```python
from build123d import *

# Parameters (mm, degrees)
SKETCH_1_W           = 76.5
SKETCH_1_H           = 50.4
SKETCH_1_W_2         = 72.5
SKETCH_1_H_2         = 46.4
EXTRUDE_1_DEPTH      = 3
SKETCH_2_W           = 26.5
SKETCH_2_H           = 2
SKETCH_2_W_2         = 2
SKETCH_2_H_2         = 7
EXTRUDE_2_DEPTH      = 3
EXTRUDE_4_DEPTH      = 2
EXTRUDE_4_DEPTH_BACK = 18
SKETCH_3_W           = 76.541364071
SKETCH_3_H           = 20
SKETCH_3_R           = 2.7
FILLET_1_R           = 3
CUT_EXTRUDE_1_DEPTH  = 18
SKETCH_5_W           = 42.5
SKETCH_5_H           = 5
EXTRUDE_5_DEPTH      = 2
EXTRUDE_6_DEPTH      = 2
SKETCH_7_W           = 26.5
SKETCH_7_H           = 2
EXTRUDE_7_DEPTH      = 2
SKETCH_8_W           = 67.5
SKETCH_8_H           = 2
EXTRUDE_8_DEPTH      = 10


with BuildPart() as part:
    # 草图1 → 凸台-拉伸1 (new body)
    with BuildSketch(Plane(origin=(0, 0, 0), x_dir=(0, 0, -1), z_dir=(1, 0, 0))):
        with Locations((36.25, 23.2)):
            Rectangle(SKETCH_1_W, SKETCH_1_H)
        with Locations((36.25, 23.2)):
            Rectangle(SKETCH_1_W_2, SKETCH_1_H_2, mode=Mode.SUBTRACT)
    extrude(amount=EXTRUDE_1_DEPTH)

    # 草图2 → 凸台-拉伸2 (add)
    with BuildSketch(Plane(origin=(3, 0, 0), x_dir=(0, 0, -1), z_dir=(1, 0, 0))):
        with Locations((36.25, -1)):
            Rectangle(SKETCH_2_W, SKETCH_2_H)
        Polygon((-2, -2), (0, -2), (5, -2), (5, 0), (0, 0), (0, 28), (-2, 28), align=None)
        Polygon((74.5, -2), (72.5, -2), (67.5, -2), (67.5, 0), (72.5, 0), (72.5, 8), (74.5, 8), align=None)
        Polygon((-2, 48.4), (5, 48.4), (5, 46.4), (0, 46.4), (0, 41.4), (-2, 41.4), (-2, 46.4), align=None)
        with Locations((73.5, 44.9)):
            Rectangle(SKETCH_2_W_2, SKETCH_2_H_2)
    extrude(amount=EXTRUDE_2_DEPTH)

    # 草图3 → 凸台-拉伸4 (add, two sides: drawn at the far end of the back side and taken through both)
    with BuildSketch(Plane.ZY.offset(-EXTRUDE_4_DEPTH_BACK)):
        with Locations((-36.229317964, 58.4)):
            Rectangle(SKETCH_3_W, SKETCH_3_H)
        with Locations((-59.5, 53.4)):
            Circle(SKETCH_3_R, mode=Mode.SUBTRACT)
        with Locations((-12.958635929, 53.4)):
            Circle(SKETCH_3_R, mode=Mode.SUBTRACT)
        with Locations((-34.458635929, 53.4)):
            Circle(SKETCH_3_R, mode=Mode.SUBTRACT)
    extrude(amount=EXTRUDE_4_DEPTH + EXTRUDE_4_DEPTH_BACK)

    # 圆角1
    fillet_1_edges = [part.edges().sort_by_distance(p)[0] for p in [
        (18, 68.4, -36.229317964),
    ]]
    fillet(fillet_1_edges, radius=FILLET_1_R)

    # 草图4 → 切除-拉伸1 (cut)
    with BuildSketch(Plane(origin=(0, 68.4, 0), x_dir=(1, 0, 0), z_dir=(0, 1, 0))):
        with BuildLine():
            Line((7.8, 66.5), (7.8, 51.5))
            ThreePointArc((7.8, 51.5), (5.15, 48.85), (2.5, 51.5))
            Line((2.5, 51.5), (2.5, 66.5))
            ThreePointArc((2.5, 66.5), (5.15, 69.15), (7.8, 66.5))
        make_face()
        with BuildLine():
            Line((7.8, 29.958635929), (7.8, 9.958635929))
            ThreePointArc((7.8, 9.958635929), (5.15, 7.308635929), (2.5, 9.958635929))
            Line((2.5, 9.958635929), (2.5, 29.958635929))
            ThreePointArc((2.5, 29.958635929), (5.15, 32.608635929), (7.8, 29.958635929))
        make_face()
    extrude(amount=-CUT_EXTRUDE_1_DEPTH, mode=Mode.SUBTRACT)

    # 草图5 → 凸台-拉伸5 (add)
    with BuildSketch(Plane.ZY):
        Polygon((-35.66479448, 48.4), (-36.83520552, 48.4), (-57.5, 35.174531533), (-57.5, 48.4), (-60.5, 48.4), (-60.5, 33.254531533), (-74.5, 24.294531533), (-74.5, 21.2), (2, 21.2), (2, 24.294531533), (-12, 33.254531533), (-12, 48.4), (-15, 48.4), (-15, 35.174531533), align=None)
        Polygon((-60.5, 23.2), (-72.5, 23.2), (-60.5, 30.88), align=None, mode=Mode.SUBTRACT)
        with Locations((-36.25, 25.7)):
            Rectangle(SKETCH_5_W, SKETCH_5_H, mode=Mode.SUBTRACT)
        Polygon((-12, 30.88), (0, 23.2), (-12, 23.2), align=None, mode=Mode.SUBTRACT)
        Polygon((-57.5, 32.8), (-36.25, 46.4), (-15, 32.8), (-15, 30.88), (-57.5, 30.88), align=None, mode=Mode.SUBTRACT)
    extrude(amount=EXTRUDE_5_DEPTH)

    # 草图6 → 凸台-拉伸6 (add)
    with BuildSketch(Plane.ZY):
        Polygon((0, 46.4), (0, 25.574531533), (2, 24.294531533), (2, 48.4), (-12, 48.4), (-12, 46.4), align=None)
        Polygon((-74.5, 48.4), (-74.5, 24.294531533), (-72.5, 25.574531533), (-72.5, 46.4), (-60.5, 46.4), (-60.5, 48.4), align=None)
        Polygon((2, -2), (2, 21.2), (0, 21.2), (0, 0), (-72.5, 0), (-72.5, 21.2), (-74.5, 21.2), (-74.5, -2), align=None)
        Polygon((-15, 46.4), (-15, 48.4), (-35.66479448, 48.4), (-32.53979448, 46.4), align=None)
        Polygon((-57.5, 46.4), (-39.96020552, 46.4), (-36.83520552, 48.4), (-57.5, 48.4), align=None)
    extrude(amount=EXTRUDE_6_DEPTH)

    # 草图7 → 凸台-拉伸7 (add)
    with BuildSketch(Plane(origin=(6, 0, 0), x_dir=(0, 0, -1), z_dir=(1, 0, 0))):
        with Locations((36.25, -1)):
            Rectangle(SKETCH_7_W, SKETCH_7_H)
    extrude(amount=EXTRUDE_7_DEPTH)

    # 草图8 → 凸台-拉伸8 (add)
    with BuildSketch(Plane(origin=(3, 0, 0), x_dir=(0, 0, -1), z_dir=(1, 0, 0))):
        with Locations((38.75, 47.4)):
            Rectangle(SKETCH_8_W, SKETCH_8_H)
    extrude(amount=EXTRUDE_8_DEPTH)


solid = part.part
```
The listing builds one solid part. Answer for the finished solid, in the listing's coordinates (mm). A direction names the side the tool comes from. Give positions to 0.01 mm unless a question says otherwise; leave off trailing zeros. Loops run counter-clockwise (first coordinate to the right, second up) from the corner with the lowest first, then second, coordinate; pieces in that order, holes last. Notation, with made-up numbers: M -23,37 L 10,37 A14 cw 10,62 Z; hole C 32,22.25 d3. An arc over 180 degrees is marked long. One line per item, written item: value.
1. Section C-C on x = 1.25 is taken. Determine the outline of the cut face in (y, z).
Found:
outline: M -2,-74.5 L 68.4,-74.5 L 68.4,2.04 L 48.4,2.04 L 48.4,2 L -2,2 Z; hole M 0,-72.5 L 46.4,-72.5 L 46.4,0 L 0,0 Z; hole C 53.4,-59.5 d5.4; hole C 53.4,-34.46 d5.4; hole C 53.4,-12.96 d5.4
2. For a pull along Y with two mould halves and no side action, classify faces 5 (the face through (5.21, 59.53, -7.31)), 6 (the face through (0, 30, -34)), 7 (the face through (7, 68.4, -37)) as pulls with the +Y half, pulls with the -Y half, needs draft (parallel to the pull), parting line crosses it, or undercut.
Found:
face 5: needs draft
face 6: undercut
face 7: pulls with the +Y half
3. Each of these flat-tipped pins is pushed along its axis until it touches: P1, Ø12, axis at x = 15, z = -22.5, coming from the -Y side; P2, Ø1, axis at x = 8, y = 47.5, coming from the +Z side; P3, Ø0.6, axis at y = 33.5, z = 1.5, coming from the +X side; P4, Ø1.5, axis at y = 19, z = -36, coming from the +X side. Where does it stop, or does it pass through?
Found:
P1: y = 46.4
P2: z = -5
P3: x = 3
P4: through
4. Find the intervals of material crossed by probe 1 along Y at (x, z) = (11, -59.5); probe 2 along Z at (x, y) = (6.5, 53); probe 3 along Y at (x, z) = (-0.5, -59), in increasing order.
Found:
probe 1: 46.4 to 50.7, 56.1 to 68.4
probe 2: -74.5 to -68.78, -49.22 to -37.13, -7.68 to 2.04
probe 3: -2 to 0, 21.2 to 50.75, 56.05 to 68.4
5. Section D-D on y = 62.5 is taken. Determine the outline of the cut face in (x, z), plus the area to 3 significant figures.
Found:
outline: M -2,-74.5 L 18,-74.5 L 18,2.04 L -2,2.04 Z; hole M 2.5,-66.5 A2.65 ccw 7.8,-66.5 L 7.8,-51.5 A2.65 ccw 2.5,-51.5 Z; hole M 2.5,-29.96 A2.65 ccw 7.8,-29.96 L 7.8,-9.96 A2.65 ccw 2.5,-9.96 Z
area: 1,300 mm^2
6. For faces 1 (the face through (6, 45, -73)), 2 (the face through (5, 50.4, -20)), 3 (the face through (3, 35, 1)), 4 (the face through (-1, 23.2, -66)), determine the directions among +Z, -Z, +X, -X, +Y, -Y from which every point of the face is accessible in a straight line to the end or side of a thin tool.
Found:
face 1: -Z, +X, -Y
face 2: +Y
face 3: +Z, -Z, +X
face 4: +X, -X
7. Section B-B on z = -59.5 is taken. Determine the outline of the cut face in (x, y), plus the area to 3 significant figures.
Found:
outline: M -2,-2 L 3,-2 L 3,0 L -2,0 Z; M -2,21.2 L 0,21.2 L 0,46.4 L 13,46.4 L 13,48.4 L 18,48.4 L 18,50.7 L 7.8,50.7 L 7.8,50.4 L 2.5,50.4 L 2.5,50.7 L -2,50.7 Z; M -2,56.1 L 2.5,56.1 L 2.5,68.4 L -2,68.4 Z; M 7.8,56.1 L 18,56.1 L 18,65.4 A3 ccw 15,68.4 L 7.8,68.4 Z
area: 314 mm^2
8. Section A-A on y = 11 is taken. Determine the outline of the cut face in (x, z), plus the area to 3 significant figures.
Found:
outline: M -2,-74.5 L 3,-74.5 L 3,-72.5 L -2,-72.5 Z; M -2,0 L 6,0 L 6,2 L -2,2 Z
area: 26.0 mm^2
